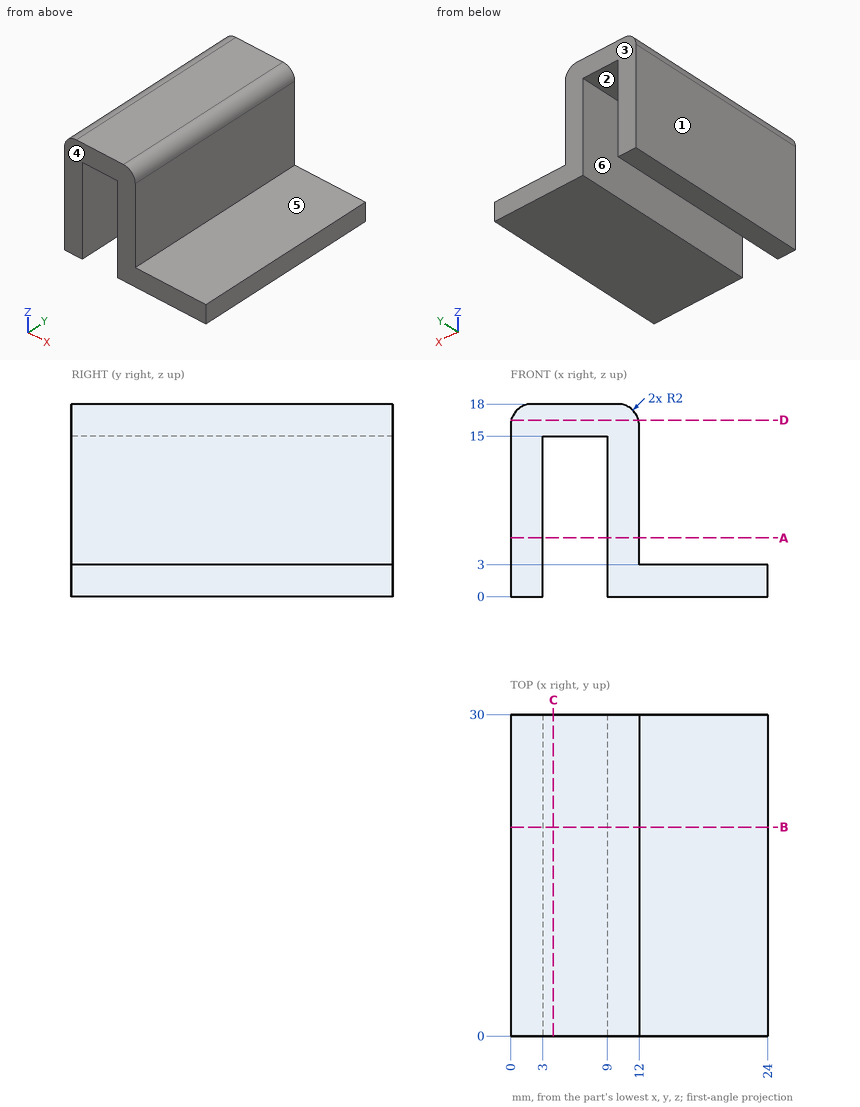
Verification items for this drawing (mm, ordinates from the low corner). A direction names the side the tool comes from. Give positions to 0.01 mm unless a question says otherwise; leave off trailing zeros. Write each loop counter-clockwise with the first axis right and the second up, starting at its lowest first coordinate (ties: lowest second). Pieces come first, ordered by that corner, then holes. Notation, with made-up numbers: (-24, 84.25) - (9, 84.25) arc R21 cw to (9, 94.25) - close; hole circle Ø1 at (32.25, -9.5). An arc over 180 degrees is marked (long way). Answer as a JSON object with one key per item and string values. Group by question number.
1) Thickness scan on probe 1 along X at (y, z) = (6.5, 4.25); probe 2 along X at (y, z) = (12.5, 2.5); probe 3 along Z at (x, y) = (8.5, 15.5). Record the ranges inside material, lowest first. Write a range as from..to.
2) Sectioned sample at C-C (x = 4). Record the cut outline in (y, z).
3) Sectioned sample at D-D (z = 16.5). Record the cut outline in (x, y).
4) Depth check by flat-ended pin: P1, Ø1, axis at y = 19.5, z = 13, coming from the +X side; P2, Ø13, axis at x = 17, y = 13.5, coming from the +Z side; P3, Ø5, axis at x = 11.5, y = 14, coming from the +Z side. Enter the tip coordinate at first touch or a pass-through.
5) Release check for a two-part mould opening along X. For the marked faces 1, 2 and 3 record: pulls with the +X half, pulls with the -X half, needs draft (parallel to the pull), parting line crosses it, or undercut.
6) Access from +Z, -Z, +X, -X, +Y, -Y to the whole of each face (thin tool, end or side, straight path). Record for the marked faces 4, 5 and 6.
7) Sectioned sample at A-A (z = 5.5). Record the cut outline in (x, y), then the cut area to 3 significant figures.
8) Sectioned sample at B-B (y = 19.5). Record the cut outline in (x, z).
Geometry results:
{
 "1": {"probe 1": "x = 0..3, 9..12", "probe 2": "x = 0..3, 9..24", "probe 3": "z = 15..18"},
 "2": {"outline": "(0, 15) - (30, 15) - (30, 18) - (0, 18) - close"},
 "3": {"outline": "(0.06, 0) - (11.94, 0) - (11.94, 30) - (0.06, 30) - close"},
 "4": {"P1": "stops at x = 12", "P2": "stops at z = 17.94", "P3": "stops at z = 18"},
 "5": {"face 1": "pulls with the -X half", "face 2": "undercut", "face 3": "needs draft"},
 "6": {"face 4": "+Z, -Z, +X, -X, -Y", "face 5": "+Z, +X, +Y, -Y", "face 6": "-Z, +Y, -Y"},
 "7": {"outline": "(0, 0) - (3, 0) - (3, 30) - (0, 30) - close; (9, 0) - (12, 0) - (12, 30) - (9, 30) - close", "area": "180 mm^2"},
 "8": {"outline": "(0, 0) - (3, 0) - (3, 15) - (9, 15) - (9, 0) - (24, 0) - (24, 3) - (12, 3) - (12, 16) arc R2 ccw to (10, 18) - (2, 18) arc R2 ccw to (0, 16) - close"}
}
